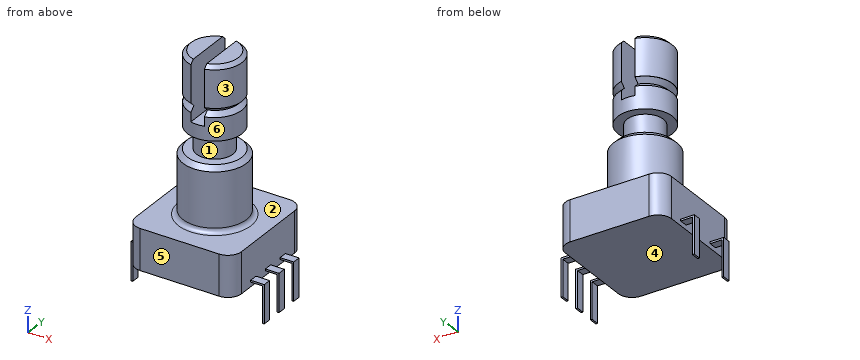
```python
from build123d import *

# Parameters (mm, degrees)
SKETCH_W             = 11.7
SKETCH_H             = 12
PAD_DEPTH            = 4.5
SKETCH001_R          = 3.5
PAD001_DEPTH         = 7
SKETCH002_R          = 2
PAD002_DEPTH         = 2.5
SKETCH004_R          = 3
PAD003_DEPTH         = 8
SKETCH005_W          = 1
SKETCH005_H          = 0.202996
POCKET_DEPTH         = 6.5
CHAMFER_SIZE         = 0.4
CHAMFER001_SIZE      = 0.5
FILLET_R             = 0.5
FILLET001_R          = 1.5
PAD004_DEPTH         = 0.45
PAD004_DEPTH_BACK    = 0.45
LINEARPATTERN_COUNT  = 3
LINEARPATTERN_PITCH  = 2.5
POCKET001_DEPTH      = 1
POCKET001_DEPTH_BACK = 1


with BuildPart() as part:
    # Sketch → Pad (new body)
    with BuildSketch(Plane.XY):
        with Locations((5.85, 6)):
            Rectangle(SKETCH_W, SKETCH_H)
    extrude(amount=PAD_DEPTH)

    # Sketch001 (on Face6 of Pad) → Pad001 (join)
    with BuildSketch(Plane.XY.offset(4.5)):
        with Locations((5.823836, 6)):
            Circle(SKETCH001_R)
    extrude(amount=PAD001_DEPTH)

    # Sketch002 (on Face8 of Pad001) → Pad002 (join)
    with BuildSketch(Plane.XY.offset(11.5)):
        with Locations((5.823836, 6)):
            Circle(SKETCH002_R)
    extrude(amount=PAD002_DEPTH)

    # Sketch004 (on Face10 of Pad002) → Pad003 (join)
    with BuildSketch(Plane.XY.offset(14)):
        with Locations((5.823836, 6)):
            Circle(SKETCH004_R)
    extrude(amount=PAD003_DEPTH)

    # Sketch005 (on DatumPlane) → Groove (revolve, cut)
    with BuildSketch(Plane(origin=(5.85, 6, 2.25), x_dir=(0, 0, -1), z_dir=(1, 0, 0))):
        Polygon((-15.25, 3), (-14.75, 2.5), (-14.25, 3), align=None)
        with Locations((-14.75, 3.101498)):
            Rectangle(SKETCH005_W, SKETCH005_H)
    revolve(axis=Axis((5.85, 6, 2.25), (0, 0, -1)), mode=Mode.SUBTRACT)

    # Sketch006 (on Face17 of Groove) → Pocket (cut)
    with BuildSketch(Plane.XY.offset(22)):
        with BuildLine():
            Line((5.073836, 8.904738), (5.073836, 3.095262))
            ThreePointArc((5.073836, 3.095262), (5.823836, 3), (6.573836, 3.095262))
            Line((6.573836, 3.095262), (6.573836, 8.904738))
            ThreePointArc((6.573836, 8.904738), (5.823836, 9), (5.073836, 8.904738))
        make_face()
    extrude(amount=-POCKET_DEPTH, mode=Mode.SUBTRACT)

    # Chamfer
    chamfer_edges = [part.edges().sort_by_distance(p)[0] for p in [
        (8.195544, 7.837117, 22),
        (8.195544, 4.162883, 22),
        (2.823836, 6, 22),
    ]]
    chamfer(chamfer_edges, length=CHAMFER_SIZE)

    # Chamfer001
    chamfer001_edges = [part.edges().sort_by_distance(p)[0] for p in [
        (2.323836, 6, 11.5),
    ]]
    chamfer(chamfer001_edges, length=CHAMFER001_SIZE)

    # Fillet
    fillet_edges = [part.edges().sort_by_distance(p)[0] for p in [
        (2.323836, 6, 4.5),
    ]]
    fillet(fillet_edges, radius=FILLET_R)

    # Fillet001
    fillet001_edges = [part.edges().sort_by_distance(p)[0] for p in [
        (11.7, 0, 2.25),
        (11.7, 12, 2.25),
        (0, 12, 2.25),
        (0, 0, 2.25),
    ]]
    fillet(fillet001_edges, radius=FILLET001_R)

    # Sketch007 (on DatumPlane) → Pad004 (join, two sides)
    with BuildSketch(Plane(origin=(5.85, 3.5, 2.25), x_dir=(1, 0, 0), z_dir=(0, -1, 0))) as pad004_sk:
        Polygon((5.85, -1.55), (5.85, -1.75), (7.15, -1.75), (7.15, -5.75), (7.35, -5.75), (7.35, -1.75), (7.35, -1.55), align=None)
        Polygon((-5.85, -1.55), (-5.85, -1.75), (-7.15, -1.75), (-7.15, -5.75), (-7.35, -5.75), (-7.35, -1.75), (-7.35, -1.55), align=None)
    pad004 = extrude(amount=PAD004_DEPTH) + extrude(pad004_sk.sketch, amount=-PAD004_DEPTH_BACK)

    # LinearPattern: Pad004 ×3
    with Locations(*[(0, i * LINEARPATTERN_PITCH, 0) for i in range(1, LINEARPATTERN_COUNT)]):
        add(pad004)

    # Sketch008 (on DatumPlane) → Pocket001 (cut, two sides)
    with BuildSketch(Plane(origin=(5.85, 6, 2.25), x_dir=(0, 0, -1), z_dir=(0, -1, 0))) as pocket001_sk:
        Polygon((1.55, -7.35), (1.55, -5.85), (1.75, -5.85), (1.75, -7.15), (5.75, -7.15), (5.75, -7.35), align=None)
    extrude(amount=-POCKET001_DEPTH, mode=Mode.SUBTRACT)
    extrude(pocket001_sk.sketch, amount=POCKET001_DEPTH_BACK, mode=Mode.SUBTRACT)


solid = part.part
```
The model under review builds one solid part; all positions refer to its coordinate system, in mm. Face numbers are marked on the shaded views. A direction names the side the tool comes from. Round coordinates to 2 decimals unless told otherwise and drop trailing zeros. Write each loop counter-clockwise with the first axis right and the second up, starting at its lowest first coordinate (ties: lowest second). Pieces come first, ordered by that corner, then holes. Notation, with made-up numbers: (55.25, 77) - (112.25, 77) arc R37 cw to (112.25, 115) - close; hole circle Ø6 at (30, -36.75). An arc over 180 degrees is marked (long way). Use one line per item in the form item = value.
Q1. Consider section D-D (z = 16). State the section outline as (x, y) points, and give its area (3 significant figures).
Answer key:
outline = (5.07, 3.1) - (5.07, 8.9) arc R3 ccw to start; (6.57, 3.1) arc R3 ccw to (6.57, 8.9) - close
area = 19.4 mm2
Q2. Draft analysis for pull direction X (two halves, no side actions). For the marked faces 4, 5 and 6, state which applies: +X half, -X half, draft (parallel to the pull), parting line (faces both ways), or undercut.
Answer key:
face_4 = undercut
face_5 = draft
face_6 = parting line
Q3. Consider section C-C (z = 3.5). State the section outline as (x, y) points.
Answer key:
outline = (0, 1.5) arc R1.5 ccw to (1.5, 0) - (10.2, 0) arc R1.5 ccw to (11.7, 1.5) - (11.7, 10.5) arc R1.5 ccw to (10.2, 12) - (1.5, 12) arc R1.5 ccw to (0, 10.5) - close
Q4. Tool access review of the marked faces 1, 2 and 3: name each direction out of +Z, -Z, +X, -X, +Y, -Y from which nothing blocks a thin tool from reaching the whole face with its end or side.
Answer key:
face_1 = none
face_2 = +Z
face_3 = +Z, +X
Q5. Insertion check: pin 1 Ø6 at (x, y) = (8, 2) entering from -Z; pin 2 Ø0.5 at (x, y) = (12.5, 3.5) entering from -Z; pin 3 Ø0.5 at (x, y) = (12.5, 3.5) entering from +Z; pin 4 Ø1.2 at (x, z) = (-0.5, -2) entering from -Y. Each pin has a flat end and moves straight along its axis. Give the tip position at first contact, or say it passes through.
Answer key:
pin_1 = 0
pin_2 = 0.5
pin_3 = 0.7
pin_4 = through
Q6. For line 1 (Z direction, x = 8, y = 7.5); line 2 (X direction, y = 6.75, z = 2.25); line 3 (Z direction, x = 0.75, y = 2.25), list the stretches that pass through material, from the lowest coordinate up. Write a range as [from, to].
Answer key:
line_1 = [0, 11.5], [14, 16.88], [17.12, 21.96]
line_2 = [0, 11.7]
line_3 = [0, 4.5]
Q7. Consider section B-B (z = -0.75). State the section outline as (x, y) points, and give its area (3 significant figures).
Answer key:
outline = (-1.5, 3.05) - (-1.3, 3.05) - (-1.3, 3.95) - (-1.5, 3.95) - close; (-1.5, 8.05) - (-1.3, 8.05) - (-1.3, 8.95) - (-1.5, 8.95) - close; (13, 3.05) - (13.2, 3.05) - (13.2, 3.95) - (13, 3.95) - close; (13, 5.55) - (13.2, 5.55) - (13.2, 6.45) - (13, 6.45) - close; (13, 8.05) - (13.2, 8.05) - (13.2, 8.95) - (13, 8.95) - close
area = 0.900 mm2
Q8. Consider section A-A (x = -0.5). State the section outline as (y, z) points, and give its area (3 significant figures).
Answer key:
outline = (3.05, 0.5) - (3.95, 0.5) - (3.95, 0.7) - (3.05, 0.7) - close; (8.05, 0.5) - (8.95, 0.5) - (8.95, 0.7) - (8.05, 0.7) - close
area = 0.360 mm2
